Geometry check sheet. Reference: the model listing, model coordinates, mm. Coordinates: 2 decimals unless noted, no trailing zeros. Loops run counter-clockwise (first coordinate to the right, second up) from the corner with the lowest first, then second, coordinate; pieces in that order, holes last. Notation, with made-up numbers: (-25, -11) - (25, -11) arc R7 cw to (25, -7) - close; hole circle Ø9 at (-18, -17.5). An arc over 180 degrees is marked (long way). Write each question's results on one line, items separated by ' | '. Start each with the question number.
(1) Sectioned sample at C-C (z = -0.5). Enter the section's corners in (x, y), plus the area to 3 significant figures.
(2) Mould release check, pull along X, two halves, no side actions. Record for faces 1 (the face through (1, -93, 0)), 2 (the face through (0.59, -29.46, -0.99)), 3 (the face through (-24.02, -120.61, -0.99)): pulls with the +X half, pulls with the -X half, needs draft (parallel to the pull), parting line crosses it, or undercut.
(3) Sectioned sample at B-B (y = -25). Enter the section's corners in (x, z).
(4) Sectioned sample at A-A (x = 0). Enter the section's corners in (y, z).
(5) Material ranges on probe 1 along Y at (x, z) = (0, -0.95); probe 2 along X at (y, z) = (-125, -0.5); probe 3 along X at (y, z) = (-75, -0.7), recorded low to high.
(6) Go/stop test with flat-tipped pins: pin 1 Ø8 at (x, y) = (25, -125) entering from -Z; pin 2 Ø1 at (x, z) = (32.5, -0.5) entering from +Y; pin 3 Ø0.6 at (y, z) = (-68.5, -0.5) entering from -X. Record where each tip stops, or that it passes through.
(7) Sectioned sample at D-D (x = -28). Enter the section's corners in (y, z).
from build123d import *

# Parameters (mm, degrees)
EXTRUDE_1_DEPTH   = 2
HOLE_WIZARD_M81_D = 9
CHAMFER_1_SIZE    = 2


with BuildPart() as part:
    # Эскиз1 → Бобышка-Вытянуть1 (new body)
    with BuildSketch(Plane(origin=(0, 0, 0), x_dir=(1, 0, 0), z_dir=(0, 0, -1))):
        Polygon((-50, 150), (50, 150), (50, 100), (25, 100), (25, 0), (-25, 0), (-25, 100), (-50, 100), align=None)
    extrude(amount=EXTRUDE_1_DEPTH)

    # Отверстие с зазором M81 (through all)
    with Locations(Plane(origin=(0, 0, -2), x_dir=(1, 0, 0), z_dir=(0, 0, -1))):
        with Locations((0, 25), (-25, 125), (25, 125), (0, 75)):
            Hole(HOLE_WIZARD_M81_D / 2)

    # Фаска1
    chamfer_1_edges = [part.edges().sort_by_distance(p)[0] for p in [
        (-50, -100, -1),
        (-50, -150, -1),
        (50, -150, -1),
        (50, -100, -1),
        (25, 0, -1),
        (-25, 0, -1),
    ]]
    chamfer(chamfer_1_edges, length=CHAMFER_1_SIZE)


solid = part.part
Outcome:
1) outline: (-50, -148) - (-48, -150) - (48, -150) - (50, -148) - (50, -102) - (48, -100) - (25, -100) - (25, -2) - (23, 0) - (-23, 0) - (-25, -2) - (-25, -100) - (-48, -100) - (-50, -102) - close; hole circle Ø9 at (-25, -125); hole circle Ø9 at (0, -75); hole circle Ø9 at (0, -25); hole circle Ø9 at (25, -125) | area: 9,730 mm2
2) face 1: needs draft | face 2: undercut | face 3: undercut
3) outline: (-25, -2) - (-4.5, -2) - (-4.5, 0) - (-25, 0) - close; (4.5, -2) - (25, -2) - (25, 0) - (4.5, 0) - close
4) outline: (-150, -2) - (-79.5, -2) - (-79.5, 0) - (-150, 0) - close; (-70.5, -2) - (-29.5, -2) - (-29.5, 0) - (-70.5, 0) - close; (-20.5, -2) - (0, -2) - (0, 0) - (-20.5, 0) - close
5) probe 1: y = -150 to -79.5, -70.5 to -29.5, -20.5 to 0 | probe 2: x = -50 to -29.5, -20.5 to 20.5, 29.5 to 50 | probe 3: x = -25 to -4.5, 4.5 to 25
6) pin 1: passes through | pin 2: stops at y = -100 | pin 3: stops at x = -25
7) outline: (-150, -2) - (-128.35, -2) - (-128.35, 0) - (-150, 0) - close; (-121.65, -2) - (-100, -2) - (-100, 0) - (-121.65, 0) - close
